Check sheet for the modelled part. Datum: model origin and axes. Units: mm. Face numbers are marked on the shaded views. A direction names the side the tool comes from. Round coordinates to 2 decimals unless told otherwise and drop trailing zeros. Loops run counter-clockwise (first coordinate to the right, second up) from the corner with the lowest first, then second, coordinate; pieces in that order, holes last. Notation, with made-up numbers: (80, -19) - (139, -19) arc R28 ccw to (139, 3) - close; hole circle Ø8 at (-7.5, 37.5). An arc over 180 degrees is marked (long way). Put each result on its own line as item: value.
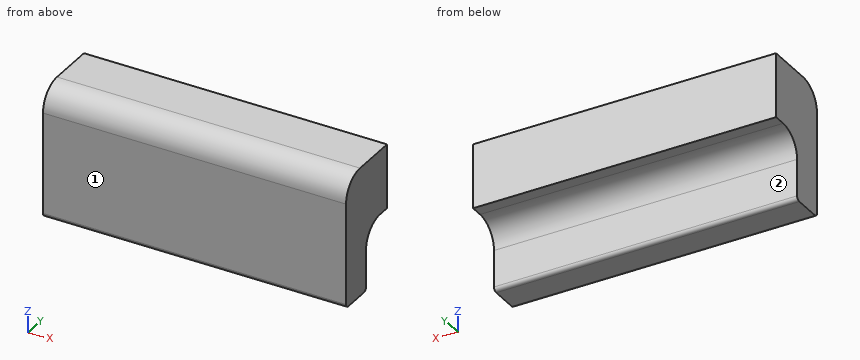
```python
from build123d import *

# Parameters (mm, degrees)
PAD_DEPTH = 80
FILLET_R  = 1


with BuildPart() as part:
    # Sketch → Pad (new body)
    with BuildSketch(Plane.YZ):
        with BuildLine():
            Line((-9.5, 0), (-18.5, 0))
            Line((-18.5, 0), (-18.5, 27.7))
            ThreePointArc((-12.2, 34), (-16.654773, 32.154773), (-18.5, 27.7))
            Line((-12.2, 34), (0, 34))
            Line((0, 34), (0, 17))
            Line((-3.2, 17), (0, 17))
            ThreePointArc((-3.2, 17), (-7.654773, 15.154773), (-9.5, 10.7))
            Line((-9.5, 0), (-9.5, 10.7))
        make_face()
    extrude(amount=PAD_DEPTH)

    # Fillet
    fillet_edges = [part.edges().sort_by_distance(p)[0] for p in [
        (40, -18.5, 0),
        (40, -9.5, 0),
    ]]
    fillet(fillet_edges, radius=FILLET_R)


solid = part.part
```
Item 1: Section check A-A on x = 53.5. Enter the section's corners in (y, z), then the cut area to 3 significant figures.
Filled sheet:
outline: (-18.5, 1) arc R1 ccw to (-17.5, 0) - (-10.5, 0) arc R1 ccw to (-9.5, 1) - (-9.5, 10.7) arc R6.3 cw to (-3.2, 17) - (0, 17) - (0, 34) - (-12.2, 34) arc R6.3 ccw to (-18.5, 27.7) - close
area: 467 mm²
Item 2: Section check B-B on z = 8. Enter the section's corners in (x, y), then the cut area to 3 significant figures.
Filled sheet:
outline: (0, -18.5) - (80, -18.5) - (80, -9.5) - (0, -9.5) - close
area: 720 mm²
Item 3: Thickness scan on line 1 (Z direction, x = 34, y = -1); line 2 (Y direction, x = 6, z = 10.5); line 3 (Z direction, x = 47.5, y = -12.5). Record the ranges inside material, lowest first. Write a range as from..to.
Filled sheet:
line 1: 17..34
line 2: -18.5..-9.5
line 3: 0..33.99
Item 4: Go/stop test with flat-tipped pins: pin 1 (10.5 mm diameter, centred on x = 21, z = 5, fed in from +Y); pin 2 (2 mm diameter, centred on x = 25, z = 13, fed in from +Y); pin 3 (3.5 mm diameter, centred on x = 43.5, y = -1, fed in from -Z). Record where each tip stops, or that it passes through.
Filled sheet:
pin 1: y = -9.5
pin 2: y = -8.57
pin 3: z = 17
Item 5: Section check C-C on y = -8.75. Enter the section's corners in (x, z), then the cut area to 3 significant figures.
Filled sheet:
outline: (0, 13.68) - (80, 13.68) - (80, 34) - (0, 34) - close
area: 1,630 mm²
Item 6: Tool access check on the marked faces 1 and 2. Record the directions out of +Z, -Z, +X, -X, +Y, -Y that give a thin tool (end or side, any length) a straight path to the whole face; none if there is none.
Filled sheet:
face 1: +Z, -Z, +X, -X, -Y
face 2: -Z, +X, -X, +Y
